Autodesk Inventor part; units mm, degrees
ref_plane "YZ Plane" through (0, 0, 0) normal (1, 0, 0) x (0, 1, 0)
ref_plane "XZ Plane" through (0, 0, 0) normal (0, 1, 0) x (-1, 0, 0)
ref_plane "XY Plane" through (0, 0, 0) normal (0, 0, 1) x (1, 0, 0)
sketch "Sketch1" plane through (0, 0, 0) normal (0, 0, 1) x (1, 0, 0)
  line L0 (0, 0) -> (0, 0.35)
  line L1 (0, 0.35) -> (5, 0.35)
  line L2 (5, 0.35) -> (5, 3)
  line L3 (5, 3) -> (20, 3)
  line L4 (20, 3) -> (20, 2.5)
  line L5 (20, 2.5) -> (20.5, 2.5)
  line L6 (20.5, 2.5) -> (20.5, 3)
  line L7 (20.5, 3) -> (22, 3)
  line L8 (0, 0) -> (27, 0)
  line L9 (27, 0) -> (27, 0.35)
  line L10 (27, 0.35) -> (22, 3)
  dimension "d0" = 0.35
  dimension "d1" = 5
  dimension "d2" = 2.65
  dimension "d3" = 15
  dimension "d4" = 0.5
  dimension "d5" = 0.5
  dimension "d6" = 0.5
  dimension "d7" = 1.5
  dimension "d8" = 27
  dimension "d9" = 0.35
revolve "Revolution1" add sketch "Sketch1" angle 360 about axis through (0, 0, 0) along (1, 0, 0)
ref_plane "Work Plane1" through (27, 0, 0) normal (1, 0, 0) x (0, 0, -1)
sketch "Sketch2" plane through (27, 0, 0) normal (1, 0, 0) x (0, 0, -1)
  circle A0 centre (0, 0) radius 0.25
  dimension "d12" = 0.5
ref_plane "Work Plane2" through (0, 0, 0) normal (-1, 0, 0) x (0, 0, 1)
sketch "Sketch3" plane through (0, 0, 0) normal (-1, 0, 0) x (0, 0, 1)
  circle A0 centre (0, 0) radius 0.25
  dimension "d14" = 0.5
sketch "Sketch4" plane through (0, 0, 0) normal (0, 0, 1) x (1, 0, 0)
  line L0 (0, 0) -> (-9.8, 0)
  line L1 (-10, -0.2) -> (-10, -10)
  line L2 (26.9718, 0) -> (36.7718, 0)
  line L3 (36.9718, -0.2) -> (36.9718, -10)
  arc A0 (-9.8, 0) -> (-10, -0.2) centre (-9.8, -0.2) ccw
  arc A1 (36.9718, -0.2) -> (36.7718, 0) centre (36.7718, -0.2) ccw
  point P0 (-10, 0)
  point P1 (36.9718, 0)
  dimension "d15" = 10
  dimension "d16" = 10
  dimension "d17" = 10
  dimension "d18" = 10
  dimension "d19" = 0.2
sweep "Sweep1" add profiles "Sketch2" path "Sketch4" path curves L2 A1 L3
sweep "Sweep2" add profiles "Sketch3" path "Sketch4" path curves L0 A0 L1
equation "\"BendRadius\" = Thickness"
equation "\"BendReliefWidth\" = Thickness"
equation "\"BendReliefDepth\" = 0.5 * Thickness"
equation "\"CornerReliefSize\" = 4 * Thickness"
equation "\"MinimumRemnant\" = 2 * Thickness"
equation "\"TransitionRadius\" = BendRadius"
equation "\"JacobiRadiusSize\" = BendRadius"
equation "\"GapSize\" = Thickness"
properties part number "k50-29"
Geometry check sheet. Reference: the model listing, model coordinates, mm. Round coordinates to 2 decimals unless told otherwise and drop trailing zeros. Loops run counter-clockwise (first coordinate to the right, second up) from the corner with the lowest first, then second, coordinate; pieces in that order, holes last. Notation, with made-up numbers: M 2.5,-26.75 L 47.5,-26.75 A28 cw 47.5,6.25 Z; hole C -17,4 d1. An arc over 180 degrees is marked long. Return JSON: item names as keys, results as strings. Group by question number.
(1) Go/stop test with flat-tipped pins: pin 1 (3 mm diameter, centred on x = 28, y = -1, fed in from +Z); pin 2 (5 mm diameter, centred on x = 30, y = -3, fed in from +Z); pin 3 (1.5 mm diameter, centred on x = 6.5, y = -2.5, fed in from +Z). Record where each tip stops, or that it passes through.
(2) Section check B-B, the plane y = -6. Enter the section's corners in (x, z).
(3) Section check A-A, the plane x = 12. Enter the section's corners in (y, z).
(4) Scan lines: line 1 along X through (y, z) = (-1.75, 0.1); line 2 along X through (y, z) = (0, 2.55); line 3 along X through (y, z) = (-1.75, 2.2). Record each from-to range of solid material in increasing order. Write a range as [from, to].
Data:
{
 "1": {"pin 1": "z = 0.45", "pin 2": "through", "pin 3": "z = 2.44"},
 "2": {"outline": "C -10,0 d0.5; C 36.97,0 d0.5"},
 "3": {"outline": "C 0,0 d6"},
 "4": {"line 1": "[-10.23, -9.77], [5, 24.35], [36.74, 37.2]", "line 2": "[5, 20], [20.5, 22.85]", "line 3": "[5, 20], [20.5, 22.36]"}
}
